```python
from build123d import *

# Parameters (mm, degrees)
SKETCH1_W                    = 30
SKETCH1_H                    = 800
BASE_FLANGE1_DEPTH           = 2
EDGE_FLANGE1_STRIP_W         = 9.4732
EDGE_FLANGE1_STRIP_H         = 2
EDGE_FLANGE1_STRIP_CUT_DEPTH = 800
EDGE_FLANGE1_DEPTH           = 800
EDGE_FLANGE2_STRIP_W         = 9.4732
EDGE_FLANGE2_STRIP_H         = 2
EDGE_FLANGE2_STRIP_CUT_DEPTH = 800
EDGE_FLANGE2_DEPTH           = 800
SKETCH12_R                   = 3
CUT_EXTRUDE1_DEPTH           = 401.562105047


# Sheet-metal steps are written as plain solids
with BuildPart() as part:
    # Sketch1 → Base-Flange1 (new body)
    with BuildSketch(Plane.XY):
        Rectangle(SKETCH1_W, SKETCH1_H)
    extrude(amount=-BASE_FLANGE1_DEPTH)

    # Edge-Flange1 strip (across the edge) → Edge-Flange1 strip cut (cut)
    with BuildSketch(Plane(origin=(15, -400, 0), x_dir=(-1, 0, 0), z_dir=(0, 1, 0))):
        with Locations((-2, -1)):
            Rectangle(EDGE_FLANGE1_STRIP_W, EDGE_FLANGE1_STRIP_H)
    extrude(amount=EDGE_FLANGE1_STRIP_CUT_DEPTH, mode=Mode.SUBTRACT)

    # Edge-Flange1 section (across the edge) → Edge-Flange1 (add)
    with BuildSketch(Plane(origin=(15, -400, 0), x_dir=(-1, 0, 0), z_dir=(0, 1, 0))):
        with BuildLine():
            Line((0, 0.7366), (0, 13))
            Line((0, 13), (2, 13))
            Line((2, 13), (2, 0.7366))
            ThreePointArc((2, 0.7366), (2.215745145, 0.215745145), (2.7366, 0))
            Line((2.7366, 0), (2.7366, -2))
            ThreePointArc((2.7366, -2), (0.801531583, -1.198468417), (0, 0.7366))
        make_face()
    extrude(amount=EDGE_FLANGE1_DEPTH)

    # Edge-Flange2 strip (across the edge) → Edge-Flange2 strip cut (cut)
    with BuildSketch(Plane(origin=(13, -400, 13), x_dir=(0, 0, -1), z_dir=(0, 1, 0))):
        with Locations((-2, -1)):
            Rectangle(EDGE_FLANGE2_STRIP_W, EDGE_FLANGE2_STRIP_H)
    extrude(amount=EDGE_FLANGE2_STRIP_CUT_DEPTH, mode=Mode.SUBTRACT)

    # Edge-Flange2 section (across the edge) → Edge-Flange2 (add)
    with BuildSketch(Plane(origin=(13, -400, 13), x_dir=(0, 0, -1), z_dir=(0, 1, 0))):
        with BuildLine():
            Line((0, 0.7366), (0, 28))
            Line((0, 28), (2, 28))
            Line((2, 28), (2, 0.7366))
            ThreePointArc((2, 0.7366), (2.215745145, 0.215745145), (2.7366, 0))
            Line((2.7366, 0), (2.7366, -2))
            ThreePointArc((2.7366, -2), (0.801531583, -1.198468417), (0, 0.7366))
        make_face()
    extrude(amount=EDGE_FLANGE2_DEPTH)

    # Sketch12 → Cut-Extrude1 (cut, through all)
    with BuildSketch(Plane(origin=(0, 0, -2), x_dir=(-1, 0, 0), z_dir=(0, 0, -1))):
        with Locations(Location((9.26, 380, 0), (0, 0, 90))):
            Circle(SKETCH12_R)
        with Locations(Location((9.26, 0, 0), (0, 0, 90))):
            Circle(SKETCH12_R)
        with Locations(Location((9.26, -380, 0), (0, 0, 90))):
            Circle(SKETCH12_R)
    extrude(amount=-CUT_EXTRUDE1_DEPTH, mode=Mode.SUBTRACT)


solid = part.part
```
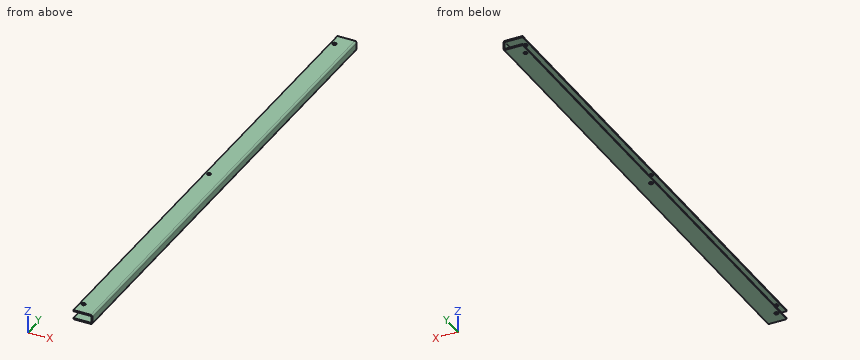
The model under review builds one solid part; all positions refer to its coordinate system, in mm. Coordinates: 2 decimals unless noted, no trailing zeros. Write each loop counter-clockwise with the first axis right and the second up, starting at its lowest first coordinate (ties: lowest second). Pieces come first, ordered by that corner, then holes.
1) We need section B-B on y = 198.5. State the section outline as (x, z) points, then the cut area to 3 significant figures.
2) We need section A-A on x = -0.5. State the section outline as (y, z) points.
3) We need section C-C on z = 7.5. State the section outline as (x, y) points.
4) Clearance check with flat-ended pins moving along their axes: pin 1 Ø1 at (y, z) = (89, 9) entering from -X; pin 2 Ø5.5 at (x, y) = (-9.26, -380) entering from +Z; pin 3 Ø7 at (x, y) = (-9.26, 0) entering from -Z. State where each tip first meets the part, or that it passes through.
5) To check wall thickness, follow probe 1 along Z at (x, y) = (-3.25, 260.5); probe 2 along X at (y, z) = (192, 4.25); probe 3 along X at (y, z) = (380, 12.2). State the ranges of each line that lie inside material, in increasing order.
Answer list:
1. outline: (-15, -2) - (12.26, -2) arc R2.74 ccw to (15, 0.74) - (15, 10.26) arc R2.74 ccw to (12.26, 13) - (-15, 13) - (-15, 11) - (12.26, 11) arc R0.74 cw to (13, 10.26) - (13, 0.74) arc R0.74 cw to (12.26, 0) - (-15, 0) - close
1. area: 139 mm2
2. outline: (-400, -2) - (400, -2) - (400, 0) - (-400, 0) - close; (-400, 11) - (400, 11) - (400, 13) - (-400, 13) - close
3. outline: (13, -400) - (15, -400) - (15, 400) - (13, 400) - close
4. pin 1: stops at x = 13
4. pin 2: passes through
4. pin 3: stops at z = -2
5. probe 1: z = -2 to 0, 11 to 13
5. probe 2: x = 13 to 15
5. probe 3: x = -15 to -12.26, -6.26 to 14.2
